from build123d import *

# Parameters (mm, degrees)
SKETCH_1_R      = 2.5
EXTRUDE_1_DEPTH = 250


with BuildPart() as part:
    # 草图1 → 拉伸1 (new body)
    with BuildSketch(Plane.XY):
        with BuildLine():
            Line((36.486773435, 27.666621685), (39.340326826, 24.813068294))
            ThreePointArc((39.340326826, 24.813068294), (39.885221932, 24.704681919), (40.193880216, 25.166621685))
            Line((40.193880216, 25.166621685), (40.193880216, 27.586722697))
            Line((40.193880216, 27.586722697), (41.693880216, 27.586722697))
            Line((41.693880216, 27.586722697), (41.693880216, 27.086722697))
            Line((41.693880216, 27.086722697), (42.193880216, 27.086722697))
            Line((42.193880216, 27.086722697), (42.193880216, 21.686722697))
            ThreePointArc((42.193880216, 21.686722697), (41.900986997, 20.979615916), (41.193880216, 20.686722697))
            Line((41.193880216, 20.686722697), (35.793880216, 20.686722697))
            Line((35.793880216, 20.686722697), (35.793880216, 21.186722697))
            Line((35.793880216, 21.186722697), (35.293880216, 21.186722697))
            Line((35.293880216, 21.186722697), (35.293880216, 22.686722697))
            Line((35.293880216, 22.686722697), (37.713981229, 22.686722697))
            ThreePointArc((37.713981229, 22.686722697), (38.175920995, 22.995380981), (38.06753462, 23.540276088))
            Line((38.06753462, 23.540276088), (35.213981229, 26.393829479))
            ThreePointArc((35.213981229, 26.393829479), (34.88955788, 26.61060223), (34.506874448, 26.686722697))
            Line((34.506874448, 26.686722697), (29.880885985, 26.686722697))
            ThreePointArc((29.880885985, 26.686722697), (29.498202552, 26.61060223), (29.173779204, 26.393829479))
            Line((29.173779204, 26.393829479), (26.320225813, 23.540276088))
            ThreePointArc((26.320225813, 23.540276088), (26.211839437, 22.995380981), (26.673779204, 22.686722697))
            Line((26.673779204, 22.686722697), (29.093880216, 22.686722697))
            Line((29.093880216, 22.686722697), (29.093880216, 21.186722697))
            Line((29.093880216, 21.186722697), (28.593880216, 21.186722697))
            Line((28.593880216, 21.186722697), (28.593880216, 20.686722697))
            Line((28.593880216, 20.686722697), (15.793880216, 20.686722697))
            Line((15.793880216, 20.686722697), (15.793880216, 21.186722697))
            Line((15.793880216, 21.186722697), (15.293880216, 21.186722697))
            Line((15.293880216, 21.186722697), (15.293880216, 22.686722697))
            Line((15.293880216, 22.686722697), (17.713981229, 22.686722697))
            ThreePointArc((17.713981229, 22.686722697), (18.175920995, 22.995380981), (18.06753462, 23.540276088))
            Line((18.06753462, 23.540276088), (15.213981229, 26.393829479))
            ThreePointArc((15.213981229, 26.393829479), (14.88955788, 26.61060223), (14.506874448, 26.686722697))
            Line((14.506874448, 26.686722697), (9.880885985, 26.686722697))
            ThreePointArc((9.880885985, 26.686722697), (9.498202552, 26.61060223), (9.173779204, 26.393829479))
            Line((9.173779204, 26.393829479), (6.320225813, 23.540276088))
            ThreePointArc((6.320225813, 23.540276088), (6.211839437, 22.995380981), (6.673779204, 22.686722697))
            Line((6.673779204, 22.686722697), (9.093880216, 22.686722697))
            Line((9.093880216, 22.686722697), (9.093880216, 21.186722697))
            Line((9.093880216, 21.186722697), (8.593880216, 21.186722697))
            Line((8.593880216, 21.186722697), (8.593880216, 20.686722697))
            Line((8.593880216, 20.686722697), (3.193880216, 20.686722697))
            ThreePointArc((3.193880216, 20.686722697), (2.486773435, 20.979615916), (2.193880216, 21.686722697))
            Line((2.193880216, 21.686722697), (2.193880216, 27.086722697))
            Line((2.193880216, 27.086722697), (2.693880216, 27.086722697))
            Line((2.693880216, 27.086722697), (2.693880216, 27.586722697))
            Line((2.693880216, 27.586722697), (4.193880216, 27.586722697))
            Line((4.193880216, 27.586722697), (4.193880216, 25.166621685))
            ThreePointArc((4.193880216, 25.166621685), (4.5025385, 24.704681919), (5.047433607, 24.813068294))
            Line((5.047433607, 24.813068294), (7.900986997, 27.666621685))
            ThreePointArc((7.900986997, 27.666621685), (8.117759749, 27.991045034), (8.193880216, 28.373728466))
            Line((8.193880216, 28.373728466), (8.193880216, 32.999716929))
            ThreePointArc((8.193880216, 32.999716929), (8.117759749, 33.382400361), (7.900986997, 33.70682371))
            Line((7.900986997, 33.70682371), (5.047433607, 36.560377101))
            ThreePointArc((5.047433607, 36.560377101), (4.5025385, 36.668763476), (4.193880216, 36.20682371))
            Line((4.193880216, 36.20682371), (4.193880216, 33.786722697))
            Line((4.193880216, 33.786722697), (2.693880216, 33.786722697))
            Line((2.693880216, 33.786722697), (2.693880216, 34.286722697))
            Line((2.693880216, 34.286722697), (2.193880216, 34.286722697))
            Line((2.193880216, 34.286722697), (2.193880216, 39.686722697))
            ThreePointArc((2.193880216, 39.686722697), (2.486773435, 40.393829479), (3.193880216, 40.686722697))
            Line((3.193880216, 40.686722697), (8.593880216, 40.686722697))
            Line((8.593880216, 40.686722697), (8.593880216, 40.186722697))
            Line((8.593880216, 40.186722697), (9.093880216, 40.186722697))
            Line((9.093880216, 40.186722697), (9.093880216, 38.686722697))
            Line((9.093880216, 38.686722697), (6.673779204, 38.686722697))
            ThreePointArc((6.673779204, 38.686722697), (6.211839437, 38.378064414), (6.320225813, 37.833169307))
            Line((6.320225813, 37.833169307), (9.173779204, 34.979615916))
            ThreePointArc((9.173779204, 34.979615916), (9.498202552, 34.762843165), (9.880885985, 34.686722697))
            Line((9.880885985, 34.686722697), (14.506874448, 34.686722697))
            ThreePointArc((14.506874448, 34.686722697), (14.88955788, 34.762843165), (15.213981229, 34.979615916))
            Line((15.213981229, 34.979615916), (18.06753462, 37.833169307))
            ThreePointArc((18.06753462, 37.833169307), (18.175920995, 38.378064414), (17.713981229, 38.686722697))
            Line((17.713981229, 38.686722697), (15.293880216, 38.686722697))
            Line((15.293880216, 38.686722697), (15.293880216, 40.186722697))
            Line((15.293880216, 40.186722697), (15.793880216, 40.186722697))
            Line((15.793880216, 40.186722697), (15.793880216, 40.686722697))
            Line((15.793880216, 40.686722697), (28.593880216, 40.686722697))
            Line((28.593880216, 40.686722697), (28.593880216, 40.186722697))
            Line((28.593880216, 40.186722697), (29.093880216, 40.186722697))
            Line((29.093880216, 40.186722697), (29.093880216, 38.686722697))
            Line((29.093880216, 38.686722697), (26.673779204, 38.686722697))
            ThreePointArc((26.673779204, 38.686722697), (26.211839437, 38.378064414), (26.320225813, 37.833169307))
            Line((26.320225813, 37.833169307), (29.173779204, 34.979615916))
            ThreePointArc((29.173779204, 34.979615916), (29.498202552, 34.762843165), (29.880885985, 34.686722697))
            Line((29.880885985, 34.686722697), (34.506874448, 34.686722697))
            ThreePointArc((34.506874448, 34.686722697), (34.88955788, 34.762843165), (35.213981229, 34.979615916))
            Line((35.213981229, 34.979615916), (38.06753462, 37.833169307))
            ThreePointArc((38.06753462, 37.833169307), (38.175920995, 38.378064414), (37.713981229, 38.686722697))
            Line((37.713981229, 38.686722697), (35.293880216, 38.686722697))
            Line((35.293880216, 38.686722697), (35.293880216, 40.186722697))
            Line((35.293880216, 40.186722697), (35.793880216, 40.186722697))
            Line((35.793880216, 40.186722697), (35.793880216, 40.686722697))
            Line((35.793880216, 40.686722697), (41.193880216, 40.686722697))
            ThreePointArc((41.193880216, 40.686722697), (41.900986997, 40.393829479), (42.193880216, 39.686722697))
            Line((42.193880216, 39.686722697), (42.193880216, 34.286722697))
            Line((42.193880216, 34.286722697), (41.693880216, 34.286722697))
            Line((41.693880216, 34.286722697), (41.693880216, 33.786722697))
            Line((41.693880216, 33.786722697), (40.193880216, 33.786722697))
            Line((40.193880216, 33.786722697), (40.193880216, 36.20682371))
            ThreePointArc((40.193880216, 36.20682371), (39.885221932, 36.668763476), (39.340326826, 36.560377101))
            Line((39.340326826, 36.560377101), (36.486773435, 33.70682371))
            ThreePointArc((36.486773435, 33.70682371), (36.270000684, 33.382400361), (36.193880216, 32.999716929))
            Line((36.193880216, 32.999716929), (36.193880216, 28.373728466))
            ThreePointArc((36.193880216, 28.373728466), (36.270000684, 27.991045034), (36.486773435, 27.666621685))
        make_face()
        with Locations((12.193880216, 30.686722697)):
            Circle(SKETCH_1_R, mode=Mode.SUBTRACT)
        with Locations((32.193880216, 30.686722697)):
            Circle(SKETCH_1_R, mode=Mode.SUBTRACT)
        with BuildLine():
            Line((16.486773435, 27.666621685), (21.48677343, 22.66662169))
            ThreePointArc((21.48677343, 22.66662169), (22.193880211, 22.373728471), (22.900986992, 22.66662169))
            Line((22.900986992, 22.66662169), (27.900986992, 27.66662169))
            ThreePointArc((27.900986992, 27.66662169), (28.117759744, 27.991045039), (28.193880211, 28.373728471))
            Line((28.193880211, 28.373728471), (28.193880211, 32.999716923))
            ThreePointArc((28.193880211, 32.999716923), (28.117759744, 33.382400355), (27.900986992, 33.706823704))
            Line((27.900986992, 33.706823704), (22.900986992, 38.706823705))
            ThreePointArc((22.900986992, 38.706823705), (22.193880211, 38.999716923), (21.48677343, 38.706823705))
            Line((21.48677343, 38.706823705), (16.486773435, 33.70682371))
            ThreePointArc((16.486773435, 33.70682371), (16.270000684, 33.382400361), (16.193880216, 32.999716929))
            Line((16.193880216, 32.999716929), (16.193880216, 28.373728466))
            ThreePointArc((16.193880216, 28.373728466), (16.270000684, 27.991045034), (16.486773435, 27.666621685))
        make_face(mode=Mode.SUBTRACT)
    extrude(amount=EXTRUDE_1_DEPTH)


solid = part.part
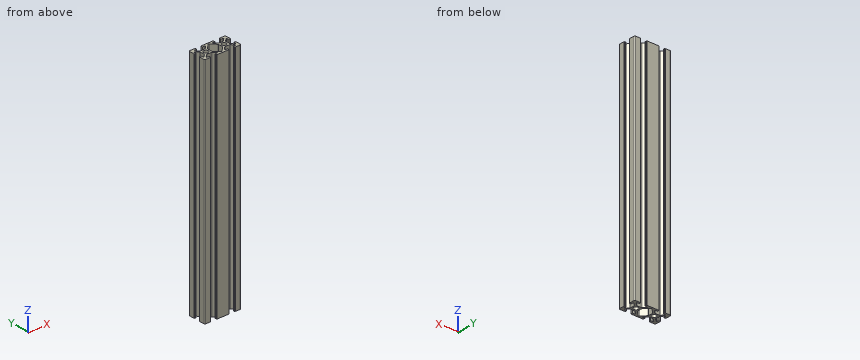
Part model, mm, in its own coordinate system. Give positions to 0.01 mm unless a question says otherwise; leave off trailing zeros. Write each question's results on one line, items separated by ' | '. Start each with the question number.
Q1. Pin check, flat tips, straight feed: P1, Ø2, axis at y = 30.5, z = 207, coming from the +X side; P2, Ø0.6, axis at y = 21, z = 94, coming from the +X side. Stop position of each tip, or through.
Q2. Wall check: L1, parallel to Y at x = 12, z = 108; L2, parallel to X at y = 21.5, z = 85.5; L3, parallel to Y at x = 28, z = 126. Give the ranges that are in metal, low to high.
Q3. Band-saw the part on A-A on z = 46. Count the separate pieces of the cut face and the enclosed holes in it, plus the area to 3 significant figures.
Results are:
1) P1: stops at x = 36.19 | P2: stops at x = 42.12
2) L1: y = 26.69 to 28.19, 33.18 to 34.69 | L2: x = 2.21 to 9.09, 15.29 to 29.09, 35.29 to 42.18 | L3: y = 20.69 to 22.69, 25.22 to 27.78, 33.59 to 36.15, 38.69 to 40.69
3) separate pieces: 1 | enclosed holes: 3 | area: 323 mm²
